Print and shaded views of the part. All mm, measured from the part's lowest x, y and z. A direction names the side the tool comes from. Give positions to 0.01 mm unless a question says otherwise; leave off trailing zeros. Loops run counter-clockwise (first coordinate to the right, second up) from the corner with the lowest first, then second, coordinate; pieces in that order, holes last. Notation, with made-up numbers: (31.25, 73.25) - (36.25, 73.25) arc R20 cw to (36.25, 81.25) - close; hole circle Ø4 at (46, -32). An arc over 180 degrees is marked (long way). Return JSON: item names as keys, results as strings.
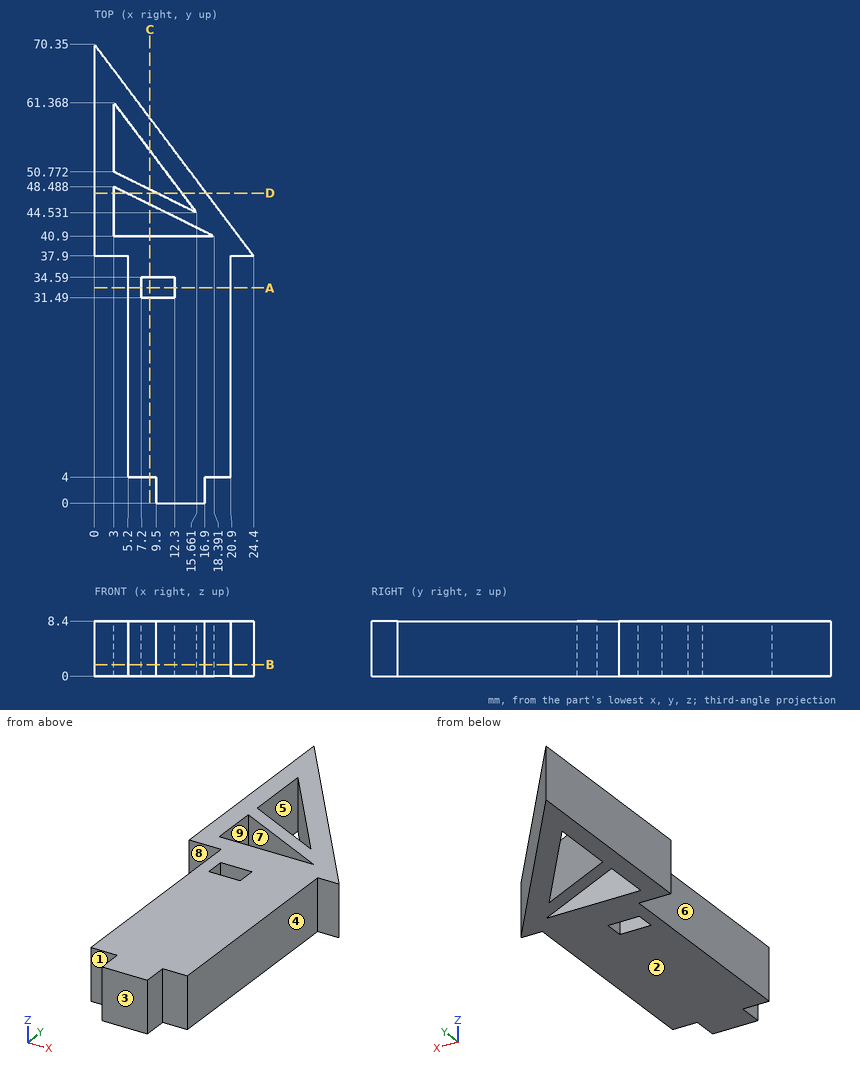
1. Cut at D-D, the plane y = 47.5. Write the cut outline in (x, z).
Values follow:
{"outline": "(0, 0) - (3, 0) - (3, 8.4) - (0, 8.4) - close; (5, 0) - (9.64, 0) - (9.64, 8.4) - (5, 8.4) - close; (13.43, 0) - (17.18, 0) - (17.18, 8.4) - (13.43, 8.4) - close"}
2. Cut at C-C, the plane x = 8.5. Write the cut outline in (y, z) (1 decimal).
Values follow:
{"outline": "(4, 0) - (31.5, 0) - (31.5, 8.4) - (4, 8.4) - close; (34.6, 0) - (40.9, 0) - (40.9, 8.4) - (34.6, 8.4) - close; (45.8, 0) - (48.1, 0) - (48.1, 8.4) - (45.8, 8.4) - close; (54.1, 0) - (59, 0) - (59, 8.4) - (54.1, 8.4) - close"}
3. Drop flat-ended pins along their axis: P1, Ø2.5, axis at x = 11, z = 3.5, coming from the +Y side (1 decimal); P2, Ø3, axis at y = 9, z = 2.5, coming from the +X side; P3, Ø4, axis at x = 8.5, z = 2.5, coming from the +Y side (1 decimal). Give the stop position or say it passes through.
Values follow:
{"P1": "stops at y = 57.4", "P2": "stops at x = 20.9", "P3": "stops at y = 61.7"}
4. Cut at A-A, the plane y = 33. Write the cut outline in (x, z).
Values follow:
{"outline": "(5.2, 0) - (7.2, 0) - (7.2, 8.4) - (5.2, 8.4) - close; (12.3, 0) - (20.9, 0) - (20.9, 8.4) - (12.3, 8.4) - close"}
5. Which spindle directions (+Z, -Z, +X, -X, +Y, -Y) get a long thin tool onto all of the face, cutting with end or side? Do the marked faces 1, 2, 3, 4 and 5. Say none if no direction does.
Values follow:
{"face 1": "+Z, -Z, -X, -Y", "face 2": "-Z, +X, -X, +Y, -Y", "face 3": "+Z, -Z, +X, -X, -Y", "face 4": "+Z, -Z, +X, -Y", "face 5": "+Z, -Z"}
6. Pull direction X, two halves, no side cores. Call the marked faces 6, 7, 8 and 9: +X half, -X half, draft (parallel to the pull), parting line (faces both ways), or undercut.
Values follow:
{"face 6": "-X half", "face 7": "undercut", "face 8": "draft", "face 9": "undercut"}
7. Cut at B-B, the plane z = 1.75. Write the cut outline in (x, y).
Values follow:
{"outline": "(0, 37.9) - (5.2, 37.9) - (5.2, 4) - (9.5, 4) - (9.5, 0) - (16.9, 0) - (16.9, 4) - (20.9, 4) - (20.9, 37.9) - (24.4, 37.9) - (0, 70.35) - close; hole (3, 40.9) - (18.39, 40.9) - (3, 48.49) - close; hole (3, 50.77) - (15.66, 44.53) - (3, 61.37) - close; hole (7.2, 31.49) - (12.3, 31.49) - (12.3, 34.59) - (7.2, 34.59) - close"}
8. Drill centre lines: probe 1 along X at (y, z) = (47.5, 6.5) (1 decimal); probe 2 along Y at (x, z) = (12.5, 5.5) (1 decimal); probe 3 along Y at (x, z) = (15, 3.5) (1 decimal). Where is each one in solid material? Low to high.
Values follow:
{"probe 1": "x = 0 to 3, 5 to 9.6, 13.4 to 17.2", "probe 2": "y = 0 to 40.9, 43.8 to 46.1, 48.7 to 53.7", "probe 3": "y = 0 to 40.9, 42.6 to 44.9, 45.4 to 50.4"}
